Answer from the drawing. Dimensions are ordinates in mm from the lowest x, y and z of the part. Round coordinates to 2 decimals unless told otherwise and drop trailing zeros. Write each loop counter-clockwise with the first axis right and the second up, starting at its lowest first coordinate (ties: lowest second). Pieces come first, ordered by that corner, then holes. Notation, with made-up numbers: (28.5, 71.25) - (57.5, 71.25) arc R33 ccw to (57.5, 99.25) - close; hole circle Ø9 at (14.25, 5.5). An arc over 180 degrees is marked (long way). Answer in a Markdown table with one row per item.
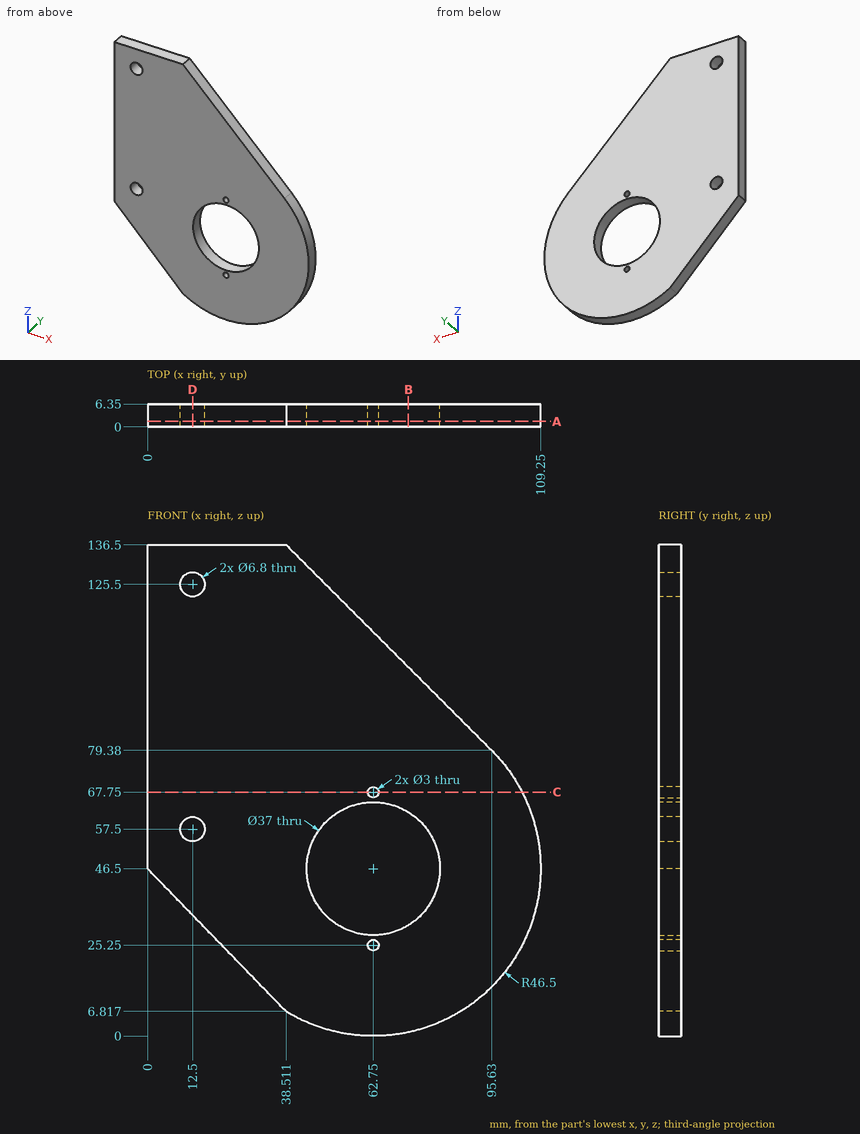
(1) Section A-A (y = 1.5) is taken. Give the vertices of the cut face in (x, z).
Checked values:
| item | result |
|---|---|
| outline | (0, 46.5) - (38.51, 6.82) arc R46.5 ccw to (95.63, 79.38) - (38.51, 136.5) - (0, 136.5) - close; hole circle Ø6.8 at (12.5, 57.5); hole circle Ø6.8 at (12.5, 125.5); hole circle Ø37 at (62.75, 46.5); hole circle Ø3 at (62.75, 25.25); hole circle Ø3 at (62.75, 67.75) |
(2) Flat-ended cylindrical pins translate along their axes: pin 1 (3 mm diameter, centred on y = 5.5, z = 78, fed in from +X); pin 2 (1.5 mm diameter, centred on y = 2, z = 37, fed in from +X). Find the tip coordinate at first contact, or state that the pin passes through.
Checked values:
| item | result |
|---|---|
| pin 1 | stops at x = 98.28 |
| pin 2 | stops at x = 108.42 |
(3) Section B-B (x = 72.5) is taken. Give the vertices of the cut face in (y, z), and give its area (3 significant figures).
Checked values:
| item | result |
|---|---|
| outline | (0, 1.03) - (6.35, 1.03) - (6.35, 30.78) - (0, 30.78) - close; (0, 62.22) - (6.35, 62.22) - (6.35, 102.51) - (0, 102.51) - close |
| area | 445 mm2 |
(4) Section D-D (x = 12.5) is taken. Give the vertices of the cut face in (y, z).
Checked values:
| item | result |
|---|---|
| outline | (0, 33.62) - (6.35, 33.62) - (6.35, 54.1) - (0, 54.1) - close; (0, 60.9) - (6.35, 60.9) - (6.35, 122.1) - (0, 122.1) - close; (0, 128.9) - (6.35, 128.9) - (6.35, 136.5) - (0, 136.5) - close |
(5) Section C-C (z = 67.75) is taken. Give the vertices of the cut face in (x, y).
Checked values:
| item | result |
|---|---|
| outline | (0, 0) - (61.25, 0) - (61.25, 6.35) - (0, 6.35) - close; (64.25, 0) - (104.11, 0) - (104.11, 6.35) - (64.25, 6.35) - close |
(6) Find the intervals of material crossed by line 1 (X direction, y = 3, z = 57.5) (1 decimal); line 2 (X direction, y = 4, z = 41) (1 decimal); line 3 (Z direction, x = 61, y = 1.25) (1 decimal), in increasing order.
Checked values:
| item | result |
|---|---|
| line 1 | x = 0 to 9.1, 15.9 to 47.9, 77.6 to 107.9 |
| line 2 | x = 5.3 to 45.1, 80.4 to 108.9 |
| line 3 | z = 0 to 28.1, 64.9 to 114 |
